```python
from build123d import *

# Parameters (mm, degrees)
PAD004_DEPTH    = 2
PAD005_DEPTH    = 3
POCKET006_DEPTH = 5
SKETCH015_R     = 1.5
POCKET007_DEPTH = 5


with BuildPart() as part:
    # Sketch011 → Pad004 (new body)
    with BuildSketch(Plane.XY):
        Polygon((-41.575623, -24.575623), (-16.575623, -24.575623), (-10, -18), (10, -18), (16.575623, -24.575623), (41.575623, -24.575623), (55, -11.151247), (55, 15.151247), (41.575623, 28.575623), (16.575623, 28.575623), (3, 15), (-3, 15), (-16.575623, 28.575623), (-41.575623, 28.575623), (-55, 15.151247), (-55, -11.151247), align=None)
    extrude(amount=PAD004_DEPTH)

    # Sketch012 (on Face18 of Pad004) → Pad005 (join)
    with BuildSketch(Plane.XY.offset(2)):
        with BuildLine():
            Line((-53, -10.32282), (-53, 14.32282))
            Line((-53, 14.32282), (-40.747196, 26.575623))
            Line((-40.747196, 26.575623), (-17.40405, 26.575623))
            Line((-17.40405, 26.575623), (-4.414214, 13.585786))
            ThreePointArc((-4.414214, 13.585786), (-3.765367, 13.152241), (-3, 13))
            Line((-3, 13), (3, 13))
            ThreePointArc((3, 13), (3.765367, 13.152241), (4.414214, 13.585786))
            Line((4.414214, 13.585786), (17.40405, 26.575623))
            Line((17.40405, 26.575623), (40.747196, 26.575623))
            Line((40.747196, 26.575623), (53, 14.32282))
            Line((53, 14.32282), (53, -10.32282))
            Line((53, -10.32282), (40.747196, -22.575623))
            Line((40.747196, -22.575623), (17.40405, -22.575623))
            Line((17.40405, -22.575623), (11.414214, -16.585786))
            ThreePointArc((11.414214, -16.585786), (10.765367, -16.152241), (10, -16))
            Line((10, -16), (-10, -16))
            ThreePointArc((-10, -16), (-10.765367, -16.152241), (-11.414214, -16.585786))
            Line((-11.414214, -16.585786), (-17.40405, -22.575623))
            Line((-17.40405, -22.575623), (-40.747196, -22.575623))
            Line((-40.747196, -22.575623), (-53, -10.32282))
        make_face()
        with BuildLine():
            Line((-51, 13.494393), (-39.918769, 24.575623))
            Line((-39.918769, 24.575623), (-18.232477, 24.575623))
            Line((-18.232477, 24.575623), (-5.828427, 12.171573))
            ThreePointArc((-5.828427, 12.171573), (-4.530734, 11.304482), (-3, 11))
            Line((-3, 11), (3, 11))
            ThreePointArc((3, 11), (4.530734, 11.304482), (5.828427, 12.171573))
            Line((5.828427, 12.171573), (18.232477, 24.575623))
            Line((18.232477, 24.575623), (39.918769, 24.575623))
            Line((39.918769, 24.575623), (51, 13.494393))
            Line((51, 13.494393), (51, -9.494393))
            Line((51, -9.494393), (39.918769, -20.575623))
            Line((39.918769, -20.575623), (18.232477, -20.575623))
            Line((18.232477, -20.575623), (12.828427, -15.171573))
            ThreePointArc((12.828427, -15.171573), (11.530734, -14.304482), (10, -14))
            Line((10, -14), (-10, -14))
            ThreePointArc((-10, -14), (-11.530734, -14.304482), (-12.828427, -15.171573))
            Line((-12.828427, -15.171573), (-18.232477, -20.575623))
            Line((-18.232477, -20.575623), (-39.918769, -20.575623))
            Line((-39.918769, -20.575623), (-51, -9.494393))
            Line((-51, -9.494393), (-51, 13.494393))
        make_face(mode=Mode.SUBTRACT)
    extrude(amount=PAD005_DEPTH)

    # Sketch014 (on Face60 of Pad005) → Pocket006 (cut)
    with BuildSketch(Plane.XY.offset(2)):
        with BuildLine():
            ThreePointArc((-11.680199, 24.776311), (-15.604738, 32.299474), (-23.127902, 28.374935))
            Line((-23.127902, 28.374935), (-24.71589, 23.323333))
            ThreePointArc((-24.71589, 23.323333), (-20.791351, 15.800169), (-13.268187, 19.724708))
            Line((-11.680199, 24.776311), (-13.268187, 19.724708))
        make_face()
        with BuildLine():
            ThreePointArc((-51.349969, 20.091476), (-58.768657, 15.972851), (-54.650031, 8.554163))
            Line((-54.650031, 8.554163), (-47.649779, 6.551855))
            ThreePointArc((-47.649779, 6.551855), (-40.231091, 10.67048), (-44.349717, 18.089168))
            Line((-51.349969, 20.091476), (-44.349717, 18.089168))
        make_face()
        with BuildLine():
            ThreePointArc((-46.279481, -20.253162), (-43.069657, -28.107908), (-35.214911, -24.898084))
            Line((-35.214911, -24.898084), (-33.002469, -19.627871))
            ThreePointArc((-33.002469, -19.627871), (-36.212293, -11.773126), (-44.067038, -14.98295))
            Line((-46.279481, -20.253162), (-44.067038, -14.98295))
        make_face()
    pocket006 = extrude(amount=POCKET006_DEPTH, mode=Mode.SUBTRACT)

    # Sketch015 (on Face4 of Pocket006) → Pocket007 (cut)
    with BuildSketch(Plane(origin=(0, 0, 0), x_dir=(1, 0, 0), z_dir=(0, 0, -1))):
        with Locations((-39.529121, 19.526524)):
            Circle(SKETCH015_R)
        with Locations((-49.976597, -13.087161)):
            Circle(SKETCH015_R)
        with Locations((-18.636831, -23.588573)):
            Circle(SKETCH015_R)
    pocket007 = extrude(amount=-POCKET007_DEPTH, mode=Mode.SUBTRACT)

    # Mirrored001: Pocket006, Pocket007 across Sketch014 V_Axis
    add(pocket006.mirror(Plane(origin=(0, 0, 2), x_dir=(0, 0, 1), z_dir=(1, 0, 0))), mode=Mode.SUBTRACT)
    add(pocket007.mirror(Plane(origin=(0, 0, 2), x_dir=(0, 0, 1), z_dir=(1, 0, 0))), mode=Mode.SUBTRACT)


with BuildPart() as part_1:
    # Body002 placement: moved
    add(part.part.moved(Location((0, 0, -42))))


solid = part_1.part
```
Design review of the part built by this model. Coordinates are the model's own, in mm. A direction names the side the tool comes from. Round coordinates to 2 decimals unless told otherwise and drop trailing zeros. Order: outer loops, then holes, each group sorted by start corner. A loop starts at its lowest first (then second) coordinate and runs counter-clockwise, first axis right, second up. Notation, with made-up numbers: (89.5, 52) - (117.5, 52) arc R22 cw to (117.5, 78) - close; hole circle Ø5 at (4.5, 85.5). An arc over 180 degrees is marked (long way). One line per question, with ' | ' between items.
Item 1: Wall thickness on line 1 (X direction, y = -1, z = -37.7); line 2 (X direction, y = 20, z = -38.25); line 3 (Z direction, x = -15, y = -11): over which ranges is each line inside the solid? List them lowest first. Write a range as [from, to].
Checks:
line 1: [-53, -51], [51, 53] | line 2: [-47.32, -44.49], [-13.18, -10.83], [10.83, 13.18], [44.49, 47.32] | line 3: [-42, -40]
Item 2: For P1, Ø2.5, axis at x = -39.53, y = -19.53, coming from the -Z side; P2, Ø2.5, axis at x = -27.5, z = -38, coming from the -Y side; P3, Ø0.9, axis at y = -4.5, z = -38.5, coming from the +X side; P4, Ø4, axis at x = 39.53, y = -19.53, coming from the -Z side, all flat-tipped, find the tip position at first contact; note any pin that passes through.
Checks:
P1: through | P2: y = -22.58 | P3: x = 53 | P4: z = -42
Item 3: Draft analysis for pull direction Y (two halves, no side actions). For faces 4 (the face through (-26, -20.576, -39)), 5 (the face through (32, 26.576, -39)), 6 (the face through (51.3, -5.9, -37)), 7 (the face through (49.22, -14.1, -38.52)), state which applies: +Y half, -Y half, draft (parallel to the pull), parting line (faces both ways), or undercut.
Checks:
face 4: undercut | face 5: +Y half | face 6: draft | face 7: -Y half
Item 4: Take a section at D-D, the plane y = -3.5. Write out the cut boundary in (x, z).
Checks:
outline: (-55, -42) - (55, -42) - (55, -40) - (53, -40) - (53, -37) - (51, -37) - (51, -40) - (-51, -40) - (-51, -37) - (-53, -37) - (-53, -40) - (-55, -40) - close
Item 5: Take a section at C-C, the plane z = -40.9. Write out the cut boundary in (x, y), then the cut area to 3 significant figures.
Checks:
outline: (-55, -11.15) - (-41.58, -24.58) - (-16.58, -24.58) - (-10, -18) - (10, -18) - (16.58, -24.58) - (41.58, -24.58) - (55, -11.15) - (55, 15.15) - (41.58, 28.58) - (16.58, 28.58) - (3, 15) - (-3, 15) - (-16.58, 28.58) - (-41.58, 28.58) - (-55, 15.15) - close; hole circle Ø3 at (-49.98, 13.09); hole circle Ø3 at (-39.53, -19.53); hole circle Ø3 at (-18.64, 23.59); hole circle Ø3 at (18.64, 23.59); hole circle Ø3 at (39.53, -19.53); hole circle Ø3 at (49.98, 13.09) | area: 5,000 mm²
Item 6: Take a section at A-A, the plane y = 16.5. Write out the cut boundary in (x, z), then the cut area to 3 significant figures.
Checks:
outline: (-53.65, -42) - (-4.5, -42) - (-4.5, -40) - (-7.33, -40) - (-7.33, -37) - (-10.16, -37) - (-10.16, -40) - (-53.65, -40) - close; (4.5, -42) - (53.65, -42) - (53.65, -40) - (10.16, -40) - (10.16, -37) - (7.33, -37) - (7.33, -40) - (4.5, -40) - close | area: 214 mm²
Item 7: Machinability: for faces 1 (the face through (47.063, 18.865, -38.521)), 2 (the face through (-53, -1, -39)), 3 (the face through (-32, 26.576, -39)), which of the approach directions +Z, -Z, +X, -X, +Y, -Y give a long, thin tool a straight path to every point of the face, cutting with its end or side? Answer none if there is none.
Checks:
face 1: +Z, +X | face 2: +Z, -X, +Y, -Y | face 3: +Z, +X, -X, +Y
Item 8: Take a section at B-B, the plane x = 28. Write out the cut boundary in (y, z).
Checks:
outline: (-24.58, -42) - (28.58, -42) - (28.58, -40) - (26.58, -40) - (26.58, -37) - (24.58, -37) - (24.58, -40) - (-20.58, -40) - (-20.58, -37) - (-22.58, -37) - (-22.58, -40) - (-24.58, -40) - close
